Design review of the part built by this model. Coordinates are the model's own, in mm. A direction names the side the tool comes from. Coordinates: 2 decimals unless noted, no trailing zeros. Order: outer loops, then holes, each group sorted by start corner. A loop starts at its lowest first (then second) coordinate and runs counter-clockwise, first axis right, second up.
from build123d import *
from build123d.topology import SkipClean

# Parameters (mm, degrees)
SKETCH1_R           = 4
BOSS_EXTRUDE1_DEPTH = 20.4
CUT_EXTRUDE3_START  = -2
CUT_EXTRUDE3_DEPTH  = 32.708900902
CUT_EXTRUDE4_START  = 2
CUT_EXTRUDE4_DEPTH  = 32.708900902
BOSS_EXTRUDE2_DEPTH = 4
CUT_EXTRUDE5_REACH  = 50.384
SKETCH7_R           = 1.6


with BuildPart() as part:
    # Sketch1 → Boss-Extrude1 (new body)
    with BuildSketch(Plane.XY):
        with BuildLine():
            Line((-2.414508498, -6.570399433), (11, -11.5))
            Line((11, -11.5), (15, -11.5))
            Line((15, -11.5), (15, 7.5))
            Line((15, 7.5), (30, 7.5))
            Line((30, 7.5), (30, 11.5))
            Line((30, 11.5), (11, 11.5))
            Line((11, 11.5), (-2.414508498, 6.570399433))
            ThreePointArc((-2.414508498, 6.570399433), (-7, 0), (-2.414508498, -6.570399433))
        make_face()
        Circle(SKETCH1_R, mode=Mode.SUBTRACT)
    extrude(amount=BOSS_EXTRUDE1_DEPTH)

    # Sketch5 → Cut-Extrude3 (cut, through all)
    with SkipClean():  # the faces are left unmerged after this step: merging them gives an invalid solid
        with BuildSketch(Plane.XY.offset(10.2).offset(CUT_EXTRUDE3_START)):
            with BuildLine():
                Line((-2.414508498, 6.570399433), (11, 11.5))
                Line((11, 11.5), (11, 2))
                Line((11, 2), (6.708203932, 2))
                ThreePointArc((6.708203932, 2), (3.135457361, 6.258506782), (-2.414508498, 6.570399433))
            make_face()
            with BuildLine():
                ThreePointArc((-2.414508498, -6.570399433), (3.135457361, -6.258506782), (6.708203932, -2))
                Line((6.708203932, -2), (11, -2))
                Line((11, -2), (11, -11.5))
                Line((11, -11.5), (-2.414508498, -6.570399433))
            make_face()
        extrude(amount=-CUT_EXTRUDE3_DEPTH, mode=Mode.SUBTRACT)

    # Sketch5_5 → Cut-Extrude4 (cut, through all)
    with SkipClean():  # the faces are left unmerged after this step: merging them gives an invalid solid
        with BuildSketch(Plane.XY.offset(10.2).offset(CUT_EXTRUDE4_START)):
            with BuildLine():
                Line((-2.414508498, 6.570399433), (11, 11.5))
                Line((11, 11.5), (11, 2))
                Line((11, 2), (6.708203932, 2))
                ThreePointArc((6.708203932, 2), (3.135457361, 6.258506782), (-2.414508498, 6.570399433))
            make_face()
            with BuildLine():
                ThreePointArc((-2.414508498, -6.570399433), (3.135457361, -6.258506782), (6.708203932, -2))
                Line((6.708203932, -2), (11, -2))
                Line((11, -2), (11, -11.5))
                Line((11, -11.5), (-2.414508498, -6.570399433))
            make_face()
        extrude(amount=CUT_EXTRUDE4_DEPTH, mode=Mode.SUBTRACT)

    # Sketch6 → Boss-Extrude2 (add)
    with SkipClean():  # the faces are left unmerged after this step: merging them gives an invalid solid
        with BuildSketch(Plane(origin=(0, 11.5, 0), x_dir=(1, 0, 0), z_dir=(0, 1, 0))):
            Polygon((14.99930592, 9.8), (30, 9.8), (30, -30.2), (14.99930592, -30.2), (11, -20.4), (11, 0), align=None)
        extrude(amount=-BOSS_EXTRUDE2_DEPTH)

    # Sketch7 → Cut-Extrude5 (cut, up to next)
    with BuildSketch(Plane(origin=(0, 11.5, 0), x_dir=(1, 0, 0), z_dir=(0, 1, 0)), mode=Mode.PRIVATE) as cut_extrude5_sk1:
        with Locations(Location((20.5, 4.8, 0), (0, 0, 270))):
            Circle(SKETCH7_R)
    cut_extrude5_tool1 = extrude(cut_extrude5_sk1.sketch, amount=-CUT_EXTRUDE5_REACH, mode=Mode.PRIVATE) & part.part
    # Sketch7 → Cut-Extrude5 (cut, up to next)
    with BuildSketch(Plane(origin=(0, 11.5, 0), x_dir=(1, 0, 0), z_dir=(0, 1, 0)), mode=Mode.PRIVATE) as cut_extrude5_sk2:
        with Locations(Location((20.5, -25.2, 0), (0, 0, 270))):
            Circle(SKETCH7_R)
    cut_extrude5_tool2 = extrude(cut_extrude5_sk2.sketch, amount=-CUT_EXTRUDE5_REACH, mode=Mode.PRIVATE) & part.part
    add(cut_extrude5_tool1.solids().sort_by_distance((20.5, 11.5, -4.8))[0], mode=Mode.SUBTRACT)
    add(cut_extrude5_tool2.solids().sort_by_distance((20.5, 11.5, 25.2))[0], mode=Mode.SUBTRACT)


solid = part.part
1. Mouldability with a two-part tool opening along Z and no side actions: class faces 5 (the flat face through (6, 0, 0)), 6 (the cylindrical face through (21.85, 9.53, 26.06)), 7 (the flat face through (11, 7, 16)) as pulls with the +Z half, pulls with the -Z half, needs draft (parallel to the pull), parting line crosses it, or undercut.
2. Insertion check: pin 1 (3.5 mm diameter, centred on x = 8, z = 2.5, fed in from -Y); pin 2 (3 mm diameter, centred on x = 10, y = -2.5, fed in from +Z); pin 3 (1.3 mm diameter, centred on x = 9, z = 18.5, fed in from +Y); pin 4 (4.5 mm diameter, centred on x = 10, z = 18, fed in from -Y). Each pin has a flat end and moves straight along its axis. Give the tip position at first contact, or say it passes through.
3. Add section B-B (x = 20.5). Give the boundary of the cut face in (y, z).
4. Add section C-C (x = 1.5). Give the boundary of the cut face in (y, z).
5. Add section D-D (y = 8.75). Give the boundary of the cut face in (x, z), and give its area (3 significant figures).
6. To check wall thickness, follow line 1 (Y direction, x = 0, z = 6.75); line 2 (Y direction, x = 18.5, z = 28.5); line 3 (X direction, y = 8.5, z = -4.8). State the ranges of each line that lie inside material, in increasing order.
7. Add section A-A (z = 19.5). Give the boundary of the cut face in (x, y).
8. For faces 1 (the flat face through (7, -7, 12.2)), 2 (the flat face through (6, 0, 20.4)), 3 (the flat face through (11, -7, 4)), 4 (the flat face through (9, 2, 4)), list the 3-axis set-ups (+Z, -Z, +X, -X, +Y, -Y) from which the entire face can be reached by the end or side of a thin tool; tool diameter is ignored.
Solution:
1. face 5: pulls with the -Z half
1. face 6: undercut
1. face 7: needs draft
2. pin 1: stops at y = -3.15
2. pin 2: stops at z = 20.4
2. pin 3: stops at y = 2
2. pin 4: stops at y = -11.5
3. outline: (7.5, -9.8) - (11.5, -9.8) - (11.5, -6.4) - (7.5, -6.4) - close; (7.5, -3.2) - (11.5, -3.2) - (11.5, 23.6) - (7.5, 23.6) - close; (7.5, 26.8) - (11.5, 26.8) - (11.5, 30.2) - (7.5, 30.2) - close
4. outline: (-8.01, 8.2) - (-6.84, 8.2) - (-6.84, 0) - (-3.71, 0) - (-3.71, 20.4) - (-6.84, 20.4) - (-6.84, 12.2) - (-8.01, 12.2) - close; (3.71, 0) - (6.84, 0) - (6.84, 8.2) - (8.01, 8.2) - (8.01, 12.2) - (6.84, 12.2) - (6.84, 20.4) - (3.71, 20.4) - close
5. outline: (3.52, 8.2) - (11, 8.2) - (11, 0) - (15, -9.8) - (30, -9.8) - (30, 30.2) - (15, 30.2) - (11, 20.4) - (11, 12.2) - (3.52, 12.2) - close; hole circle Ø3.2 at (20.5, -4.8); hole circle Ø3.2 at (20.5, 25.2)
5. area: 735 mm2
6. line 1: y = -7 to -4, 4 to 7
6. line 2: y = 7.5 to 11.5
6. line 3: x = 12.96 to 18.9, 22.1 to 30
7. outline: (6.71, -2) - (11, -2) - (11, -11.5) - (15, -11.5) - (15, 7.5) - (30, 7.5) - (30, 11.5) - (11, 11.5) - (11, 2) - (6.71, 2) arc R7 ccw (long way) to start; hole circle Ø8 at (0, 0)
8. face 1: +Z, -Y
8. face 2: +Z, +X, -X, -Y
8. face 3: -Z, -Y
8. face 4: -Z, +Y
